Could you check a few things on this model? Use its own coordinates, in mm. Face numbers are marked on the shaded views. A direction names the side the tool comes from. Coordinates: 2 decimals unless noted, no trailing zeros. Order: outer loops, then holes, each group sorted by start corner. A loop starts at its lowest first (then second) coordinate and runs counter-clockwise, first axis right, second up. Notation, with made-up numbers: (-29.75, 65) - (26.25, 65) arc R31 cw to (26.25, 103) - close; hole circle Ø10 at (56, 56). An arc over 180 degrees is marked (long way). One line per item, written item: value. Start each with the question number.
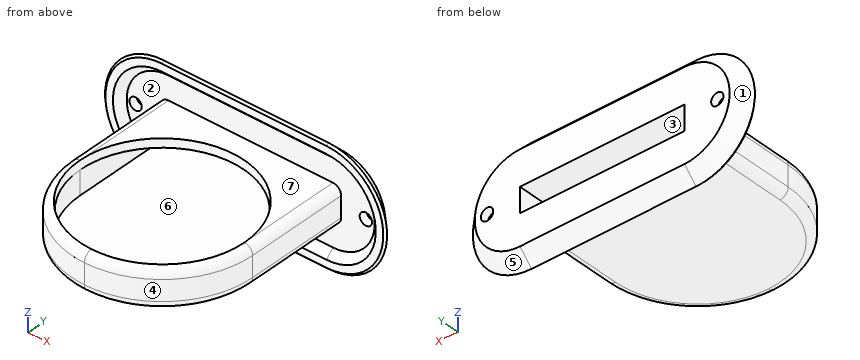
from build123d import *
from OCP.BRepFilletAPI import BRepFilletAPI_MakeChamfer

# Parameters (mm, degrees)
BOSS_EXTRU_1_DEPTH      = 3.8
BOSS_EXTRU_1_TAPER      = 45
COQUE2_DEPTH            = 1.8
COQUE2_DRAFT            = 45
CHANFREIN1_SIZE         = 1
CHANFREIN1_SIZE2        = 0.707106781
ENL_V_MAT_EXTRU_1_REACH = 39.355
ESQUISSE2_R             = 1.5
ESQUISSE3_W             = 44
ESQUISSE3_H             = 9
BOSS_EXTRU_4_DEPTH      = 47
CONG_1_R                = 22
CONG_2_R                = 2
ESQUISSE7_R             = 20
ENL_V_MAT_EXTRU_4_DEPTH = 2
ENL_V_MAT_EXTRU_4_DRAFT = -5
ENL_V_MAT_EXTRU_5_DEPTH = 6


# Read off the part's stored shape, not the designer's step: Coque2
with BuildPart() as part:
    # Esquisse1 → Boss.-Extru.1 (new body)
    with BuildSketch(Plane(origin=(0, 0, 0), x_dir=(1, 0, 0), z_dir=(0, 1, 0))):
        with BuildLine():
            ThreePointArc((-20, 14.8), (-34.8, 0), (-20, -14.8))
            Line((-20, -14.8), (20, -14.8))
            ThreePointArc((20, -14.8), (34.8, 0), (20, 14.8))
            Line((20, 14.8), (-20, 14.8))
        make_face()
    extrude(amount=BOSS_EXTRU_1_DEPTH, taper=BOSS_EXTRU_1_TAPER)


with BuildPart() as coque2_tool:
    # Coque2 outline → Coque2 (with draft: the straight prism first)
    with BuildSketch(Plane(origin=(0, 1.8, 0), x_dir=(1, 0, 0), z_dir=(0, 1, 0))):
        with BuildLine():
            Line((-20, -10.171572875), (20, -10.171572875))
            ThreePointArc((20, -10.171572875), (30.171572875, 0), (20, 10.171572875))
            Line((20, 10.171572875), (-20, 10.171572875))
            ThreePointArc((-20, 10.171572875), (-30.171572875, 0), (-20, -10.171572875))
        make_face()
    extrude(amount=-COQUE2_DEPTH)
    # Coque2: the draft: its side faces are tilted about the plane it starts from
    coque2_sides = [coque2_tool.faces().sort_by_distance(p)[0] for p in [
        (0, 0.9, 10.171572875),
        (30.171572875, 0.9, 0),
        (0, 0.9, -10.171572875),
        (-30.171572875, 0.9, 0),
    ]]
    draft(coque2_sides, Plane(origin=(0, 1.8, 0), x_dir=(1, 0, 0), z_dir=(0, 1, 0)), COQUE2_DRAFT)


with BuildPart() as part_1:
    add(part.part)

    # Coque2: cut by coque2_tool
    add(coque2_tool.part, mode=Mode.SUBTRACT)

    # Chanfrein1: one chamfer whose edges measure the first distance from different faces: ONE call of the kernel's chamfer builder (chamfer() names one face for all edges)
    chanfrein1_edges_1 = [part_1.edges().sort_by_distance(p)[0] for p in [
        (0, 0, -14.8),
        (0, 0, 14.8),
        (-34.8, 0, 0),
    ]]
    chanfrein1_side_1 = [part_1.faces().sort_by_distance(p)[0] for p in [
        (0, 0, -14.043672029),
    ]]
    chanfrein1_edges_2 = [part_1.edges().sort_by_distance(p)[0] for p in [
        (34.8, 0, 0),
    ]]
    chanfrein1_side_2 = [part_1.faces().sort_by_distance(p)[0] for p in [
        (32.9, 1.9, 0),
    ]]
    chanfrein1 = BRepFilletAPI_MakeChamfer(part_1.part.solid().wrapped)
    for e in chanfrein1_edges_1:
        chanfrein1.Add(CHANFREIN1_SIZE, CHANFREIN1_SIZE2, e.wrapped, chanfrein1_side_1[0].wrapped)  # the first distance lies on this face
    for e in chanfrein1_edges_2:
        chanfrein1.Add(CHANFREIN1_SIZE, CHANFREIN1_SIZE2, e.wrapped, chanfrein1_side_2[0].wrapped)  # the first distance lies on this face
    add(Compound.cast(chanfrein1.Shape()), mode=Mode.REPLACE)

    # Esquisse2 → Enlèv. mat.-Extru.1 (cut, up to next)
    with BuildSketch(Plane(origin=(0, 3.8, 0), x_dir=(1, 0, 0), z_dir=(0, 1, 0)), mode=Mode.PRIVATE) as enl_v_mat_extru_1_sk1:
        with Locations(Location((-28, 0, 0), (0, 0, 270))):
            Circle(ESQUISSE2_R)
    enl_v_mat_extru_1_tool1 = extrude(enl_v_mat_extru_1_sk1.sketch, amount=-ENL_V_MAT_EXTRU_1_REACH, mode=Mode.PRIVATE) & part_1.part
    # Esquisse2 → Enlèv. mat.-Extru.1 (cut, up to next)
    with BuildSketch(Plane(origin=(0, 3.8, 0), x_dir=(1, 0, 0), z_dir=(0, 1, 0)), mode=Mode.PRIVATE) as enl_v_mat_extru_1_sk2:
        with Locations(Location((28, 0, 0), (0, 0, 270))):
            Circle(ESQUISSE2_R)
    enl_v_mat_extru_1_tool2 = extrude(enl_v_mat_extru_1_sk2.sketch, amount=-ENL_V_MAT_EXTRU_1_REACH, mode=Mode.PRIVATE) & part_1.part
    add(enl_v_mat_extru_1_tool1.solids().sort_by_distance((-28, 3.8, 0))[0], mode=Mode.SUBTRACT)
    add(enl_v_mat_extru_1_tool2.solids().sort_by_distance((28, 3.8, 0))[0], mode=Mode.SUBTRACT)

    # Esquisse3 → Boss.-Extru.4 (add)
    with BuildSketch(Plane.XZ.offset(-1.8)):
        Rectangle(ESQUISSE3_W, ESQUISSE3_H)
    extrude(amount=BOSS_EXTRU_4_DEPTH)

    # Congé1
    cong_1_edges = [part_1.edges().sort_by_distance(p)[0] for p in [
        (22, -45.2, 0),
        (-22, -45.2, 0),
    ]]
    fillet(cong_1_edges, radius=CONG_1_R - 0.0001)  # a hair under: the kernel refuses the full size

    # Congé2
    cong_2_edges = [part_1.edges().sort_by_distance(p)[0] for p in [
        (-22, -10.70005, 4.5),
        (22, -10.70005, 4.5),
        (-15.556378475, -38.756378475, 4.5),
        (15.556378475, -38.756378475, 4.5),
        (22, -10.70005, -4.5),
        (-22, -10.70005, -4.5),
        (-15.556378475, -38.756378475, -4.5),
        (15.556378475, -38.756378475, -4.5),
    ]]
    fillet(cong_2_edges, radius=CONG_2_R)


with BuildPart() as enl_v_mat_extru_4_tool:
    # Esquisse7 → Enlèv. mat.-Extru.4 (with draft: the straight prism first)
    with BuildSketch(Plane.XY.offset(4.5)):
        with Locations((0, -23.2)):
            Circle(ESQUISSE7_R)
    extrude(amount=-ENL_V_MAT_EXTRU_4_DEPTH)
    # Enlèv. mat.-Extru.4: the draft: its side faces are tilted about the plane it starts from
    enl_v_mat_extru_4_sides = [enl_v_mat_extru_4_tool.faces().sort_by_distance(p)[0] for p in [
        (-20, -23.2, 3.5),
    ]]
    draft(enl_v_mat_extru_4_sides, Plane.XY.offset(4.5), ENL_V_MAT_EXTRU_4_DRAFT)


with BuildPart() as part_2:
    add(part_1.part)

    # Enlèv. mat.-Extru.4: cut by enl_v_mat_extru_4_tool
    add(enl_v_mat_extru_4_tool.part, mode=Mode.SUBTRACT)

    # Esquisse9 → Enlèv. mat.-Extru.5 (cut)
    with BuildSketch(Plane.XY.offset(2.5)):
        with BuildLine():
            Line((-20, -23.2), (-20, 3.8))
            Line((-20, 3.8), (20, 3.8))
            Line((20, 3.8), (20, -23.2))
            ThreePointArc((20, -23.2), (0, -43.2), (-20, -23.2))
        make_face()
    extrude(amount=-ENL_V_MAT_EXTRU_5_DEPTH, mode=Mode.SUBTRACT)


solid = part_2.part
Q1. We'd pull the mould along X, two halves only. Please class the marked faces 1, 2, 3 and 4: +X half, -X half, draft (parallel to the pull), parting line (faces both ways), or undercut.
Q2. I'm going to push flat-ended pins straight in: pin 1 (1.5 mm diameter, centred on y = -6, z = 0, fed in from -X); pin 2 (12 mm diameter, centred on x = -9.5, y = -17.5, fed in from -Z); pin 3 (3 mm diameter, centred on x = 25.5, z = 4.5, fed in from -Y); pin 4 (8 mm diameter, centred on y = -24, z = 11, fed in from -X). Where does each tip first touch, or does it pass through?
Q3. Which directions (+Z, -Z, +X, -X, +Y, -Y) give clear straight access to the entire face, cutting with the end or side of a thin tool? Please do the marked faces 5, 6 and 7.
Q4. I want a section at B-B on y = -1.5. Please give me the cut outline in (x, z), then the cut area to 3 significant figures.
Q5. I want a section at A-A on z = 0. State how many separate pieces and enclosed holes the cut face has, then the cut area to 3 significant figures.
Q6. If I drill on L1, parallel to X at y = 3.2, z = 0; L2, parallel to X at y = 2.7, z = 0; L3, parallel to X at y = -5, z = -1.75, over which ranges is the centre line in solid material (lowest first)?
Values follow:
1. face 1: -X half
1. face 2: undercut
1. face 3: undercut
1. face 4: +X half
2. pin 1: stops at x = -22
2. pin 2: stops at z = -4.5
2. pin 3: stops at y = 1.8
2. pin 4: passes through
3. face 5: +X, +Y
3. face 6: +Y
3. face 7: -Y
4. outline: (-22, -2.5) arc R2 ccw to (-20, -4.5) - (20, -4.5) arc R2 ccw to (22, -2.5) - (22, 2.5) arc R2 ccw to (20, 4.5) - (-20, 4.5) arc R2 ccw to (-22, 2.5) - close; hole (-20, -3.5) - (20, -3.5) - (20, 2.5) - (-20, 2.5) - close
4. area: 153 mm^2
5. separate pieces: 3
5. enclosed holes: 0
5. area: 278 mm^2
6. L1: x = -31.6 to -29.5, -26.5 to -20, 20 to 26.5, 29.5 to 31.6
6. L2: x = -32.1 to -29.5, -26.5 to -20, 20 to 26.5, 29.5 to 32.1
6. L3: x = -22 to -20, 20 to 22
